```python
from build123d import *

# Parameters (mm, degrees)
SKETCH1_W                      = 60
SKETCH1_H                      = 120
BOSS_EXTRUDE1_DEPTH            = 80
CUT_EXTRUDE2_REACH             = 106.403
SKETCH3_W                      = 50.83
SKETCH3_H                      = 25.43
CUT_EXTRUDE2_DIRECTION_2_REACH = 106.403
CUT_EXTRUDE3_REACH             = 106.403
SKETCH5_W                      = 8.9675
SKETCH5_H                      = 100
CUT_EXTRUDE3_DIRECTION_2_REACH = 106.403
CUT_EXTRUDE4_REACH             = 106.403
SKETCH6_R                      = 6.365
CUT_EXTRUDE4_DIRECTION_2_REACH = 106.403
SKETCH7_W                      = 40.03
SKETCH7_H                      = 73
SKETCH7_R                      = 2.5
SKETCH7_W_2                    = 20.03
SKETCH7_H_2                    = 40.03
BOSS_EXTRUDE2_DEPTH            = 12.5
FILLET2_R                      = 5


with BuildPart() as part:
    # Sketch1 → Boss-Extrude1 (new, symmetric)
    with BuildSketch(Plane(origin=(0, 0, 0), x_dir=(1, 0, 0), z_dir=(0, 1, 0))):
        Rectangle(SKETCH1_W, SKETCH1_H)
    extrude(amount=BOSS_EXTRUDE1_DEPTH, both=True)

    # Cut-Extrude2: up to this face of the body (flat: up to its plane)
    cut_extrude2_end = Plane(part.part.faces().sort_by_distance((0, -80, 0))[0])
    # Sketch3 → Cut-Extrude2 (cut, up to the picked face)
    with BuildSketch(Plane(origin=(0, 0, 0), x_dir=(0, 0, -1), z_dir=(0, 1, 0)), mode=Mode.PRIVATE) as cut_extrude2_sk1:
        Rectangle(SKETCH3_W, SKETCH3_H)
    cut_extrude2_tool1 = split(extrude(cut_extrude2_sk1.sketch, amount=-CUT_EXTRUDE2_REACH, mode=Mode.PRIVATE), bisect_by=cut_extrude2_end, keep=Keep.BOTH, mode=Mode.PRIVATE)
    add(cut_extrude2_tool1.solids().sort_by(Axis((0, 0, 0), (0, -1, 0)))[0], mode=Mode.SUBTRACT)

    # Cut-Extrude2 direction 2: up to this face of the body (flat: up to its plane)
    cut_extrude2_direction_2_end = Plane(part.part.faces().sort_by_distance((0, 80, 0))[0])
    # Sketch3 → Cut-Extrude2 direction 2 (cut, up to the picked face)
    with BuildSketch(Plane(origin=(0, 0, 0), x_dir=(0, 0, -1), z_dir=(0, 1, 0)), mode=Mode.PRIVATE) as cut_extrude2_direction_2_sk1:
        Rectangle(SKETCH3_W, SKETCH3_H)
    cut_extrude2_direction_2_tool1 = split(extrude(cut_extrude2_direction_2_sk1.sketch, amount=CUT_EXTRUDE2_DIRECTION_2_REACH, mode=Mode.PRIVATE), bisect_by=cut_extrude2_direction_2_end, keep=Keep.BOTH, mode=Mode.PRIVATE)
    add(cut_extrude2_direction_2_tool1.solids().sort_by(Axis((0, 0, 0), (0, 1, 0)))[0], mode=Mode.SUBTRACT)

    # Cut-Extrude3: up to this face of the body (flat: up to its plane)
    cut_extrude3_end = Plane(part.part.faces().sort_by_distance((0, 0, 60))[0])
    # Sketch5 → Cut-Extrude3 (cut, up to the picked face)
    with BuildSketch(Plane.XY, mode=Mode.PRIVATE) as cut_extrude3_sk1:
        Rectangle(SKETCH5_W, SKETCH5_H)
    cut_extrude3_tool1 = split(extrude(cut_extrude3_sk1.sketch, amount=CUT_EXTRUDE3_REACH, mode=Mode.PRIVATE), bisect_by=cut_extrude3_end, keep=Keep.BOTH, mode=Mode.PRIVATE)
    add(cut_extrude3_tool1.solids().sort_by(Axis((0, 0, 0), (0, 0, 1)))[0], mode=Mode.SUBTRACT)

    # Cut-Extrude3 direction 2: up to this face of the body (flat: up to its plane)
    cut_extrude3_direction_2_end = Plane(part.part.faces().sort_by_distance((0, 0, -60))[0])
    # Sketch5 → Cut-Extrude3 direction 2 (cut, up to the picked face)
    with BuildSketch(Plane.XY, mode=Mode.PRIVATE) as cut_extrude3_direction_2_sk1:
        Rectangle(SKETCH5_W, SKETCH5_H)
    cut_extrude3_direction_2_tool1 = split(extrude(cut_extrude3_direction_2_sk1.sketch, amount=-CUT_EXTRUDE3_DIRECTION_2_REACH, mode=Mode.PRIVATE), bisect_by=cut_extrude3_direction_2_end, keep=Keep.BOTH, mode=Mode.PRIVATE)
    add(cut_extrude3_direction_2_tool1.solids().sort_by(Axis((0, 0, 0), (0, 0, -1)))[0], mode=Mode.SUBTRACT)

    # Cut-Extrude4: up to this face of the body (flat: up to its plane)
    cut_extrude4_end = Plane(part.part.faces().sort_by_distance((30, 0, 0))[0])
    # Sketch6 → Cut-Extrude4 (cut, up to the picked face)
    with BuildSketch(Plane(origin=(0, 0, 0), x_dir=(0, 0, -1), z_dir=(1, 0, 0)), mode=Mode.PRIVATE) as cut_extrude4_sk1:
        with Locations((-39.705, -30)):
            Circle(SKETCH6_R)
    cut_extrude4_tool1 = split(extrude(cut_extrude4_sk1.sketch, amount=CUT_EXTRUDE4_REACH, mode=Mode.PRIVATE), bisect_by=cut_extrude4_end, keep=Keep.BOTH, mode=Mode.PRIVATE)
    # Sketch6 → Cut-Extrude4 (cut, up to the picked face)
    with BuildSketch(Plane(origin=(0, 0, 0), x_dir=(0, 0, -1), z_dir=(1, 0, 0)), mode=Mode.PRIVATE) as cut_extrude4_sk2:
        with Locations((-39.705, 30)):
            Circle(SKETCH6_R)
    cut_extrude4_tool2 = split(extrude(cut_extrude4_sk2.sketch, amount=CUT_EXTRUDE4_REACH, mode=Mode.PRIVATE), bisect_by=cut_extrude4_end, keep=Keep.BOTH, mode=Mode.PRIVATE)
    # Sketch6 → Cut-Extrude4 (cut, up to the picked face)
    with BuildSketch(Plane(origin=(0, 0, 0), x_dir=(0, 0, -1), z_dir=(1, 0, 0)), mode=Mode.PRIVATE) as cut_extrude4_sk3:
        with Locations(Location((39.705, -30, 0), (0, 0, 180))):
            Circle(SKETCH6_R)
    cut_extrude4_tool3 = split(extrude(cut_extrude4_sk3.sketch, amount=CUT_EXTRUDE4_REACH, mode=Mode.PRIVATE), bisect_by=cut_extrude4_end, keep=Keep.BOTH, mode=Mode.PRIVATE)
    # Sketch6 → Cut-Extrude4 (cut, up to the picked face)
    with BuildSketch(Plane(origin=(0, 0, 0), x_dir=(0, 0, -1), z_dir=(1, 0, 0)), mode=Mode.PRIVATE) as cut_extrude4_sk4:
        with Locations(Location((39.705, 30, 0), (0, 0, 180))):
            Circle(SKETCH6_R)
    cut_extrude4_tool4 = split(extrude(cut_extrude4_sk4.sketch, amount=CUT_EXTRUDE4_REACH, mode=Mode.PRIVATE), bisect_by=cut_extrude4_end, keep=Keep.BOTH, mode=Mode.PRIVATE)
    add(cut_extrude4_tool1.solids().sort_by(Axis((0, -30, 39.705), (1, 0, 0)))[0], mode=Mode.SUBTRACT)
    add(cut_extrude4_tool2.solids().sort_by(Axis((0, 30, 39.705), (1, 0, 0)))[0], mode=Mode.SUBTRACT)
    add(cut_extrude4_tool3.solids().sort_by(Axis((0, -30, -39.705), (1, 0, 0)))[0], mode=Mode.SUBTRACT)
    add(cut_extrude4_tool4.solids().sort_by(Axis((0, 30, -39.705), (1, 0, 0)))[0], mode=Mode.SUBTRACT)

    # Cut-Extrude4 direction 2: up to this face of the body (flat: up to its plane)
    cut_extrude4_direction_2_end = Plane(part.part.faces().sort_by_distance((-30, 0, 0))[0])
    # Sketch6 → Cut-Extrude4 direction 2 (cut, up to the picked face)
    with BuildSketch(Plane(origin=(0, 0, 0), x_dir=(0, 0, -1), z_dir=(1, 0, 0)), mode=Mode.PRIVATE) as cut_extrude4_direction_2_sk1:
        with Locations((-39.705, -30)):
            Circle(SKETCH6_R)
    cut_extrude4_direction_2_tool1 = split(extrude(cut_extrude4_direction_2_sk1.sketch, amount=-CUT_EXTRUDE4_DIRECTION_2_REACH, mode=Mode.PRIVATE), bisect_by=cut_extrude4_direction_2_end, keep=Keep.BOTH, mode=Mode.PRIVATE)
    # Sketch6 → Cut-Extrude4 direction 2 (cut, up to the picked face)
    with BuildSketch(Plane(origin=(0, 0, 0), x_dir=(0, 0, -1), z_dir=(1, 0, 0)), mode=Mode.PRIVATE) as cut_extrude4_direction_2_sk2:
        with Locations((-39.705, 30)):
            Circle(SKETCH6_R)
    cut_extrude4_direction_2_tool2 = split(extrude(cut_extrude4_direction_2_sk2.sketch, amount=-CUT_EXTRUDE4_DIRECTION_2_REACH, mode=Mode.PRIVATE), bisect_by=cut_extrude4_direction_2_end, keep=Keep.BOTH, mode=Mode.PRIVATE)
    # Sketch6 → Cut-Extrude4 direction 2 (cut, up to the picked face)
    with BuildSketch(Plane(origin=(0, 0, 0), x_dir=(0, 0, -1), z_dir=(1, 0, 0)), mode=Mode.PRIVATE) as cut_extrude4_direction_2_sk3:
        with Locations(Location((39.705, -30, 0), (0, 0, 180))):
            Circle(SKETCH6_R)
    cut_extrude4_direction_2_tool3 = split(extrude(cut_extrude4_direction_2_sk3.sketch, amount=-CUT_EXTRUDE4_DIRECTION_2_REACH, mode=Mode.PRIVATE), bisect_by=cut_extrude4_direction_2_end, keep=Keep.BOTH, mode=Mode.PRIVATE)
    # Sketch6 → Cut-Extrude4 direction 2 (cut, up to the picked face)
    with BuildSketch(Plane(origin=(0, 0, 0), x_dir=(0, 0, -1), z_dir=(1, 0, 0)), mode=Mode.PRIVATE) as cut_extrude4_direction_2_sk4:
        with Locations(Location((39.705, 30, 0), (0, 0, 180))):
            Circle(SKETCH6_R)
    cut_extrude4_direction_2_tool4 = split(extrude(cut_extrude4_direction_2_sk4.sketch, amount=-CUT_EXTRUDE4_DIRECTION_2_REACH, mode=Mode.PRIVATE), bisect_by=cut_extrude4_direction_2_end, keep=Keep.BOTH, mode=Mode.PRIVATE)
    add(cut_extrude4_direction_2_tool1.solids().sort_by(Axis((0, -30, 39.705), (-1, 0, 0)))[0], mode=Mode.SUBTRACT)
    add(cut_extrude4_direction_2_tool2.solids().sort_by(Axis((0, 30, 39.705), (-1, 0, 0)))[0], mode=Mode.SUBTRACT)
    add(cut_extrude4_direction_2_tool3.solids().sort_by(Axis((0, -30, -39.705), (-1, 0, 0)))[0], mode=Mode.SUBTRACT)
    add(cut_extrude4_direction_2_tool4.solids().sort_by(Axis((0, 30, -39.705), (-1, 0, 0)))[0], mode=Mode.SUBTRACT)

    # Sketch7 → Boss-Extrude2 (add, symmetric)
    with BuildSketch(Plane(origin=(0, 0, 0), x_dir=(1, 0, 0), z_dir=(0, 1, 0))):
        with Locations((-50.015, 0)):
            Rectangle(SKETCH7_W, SKETCH7_H)
        with Locations(Location((-55.015, 24, 0), (0, 0, 270))):
            Circle(SKETCH7_R, mode=Mode.SUBTRACT)
        with Locations(Location((-45.015, 24, 0), (0, 0, 270))):
            Circle(SKETCH7_R, mode=Mode.SUBTRACT)
        with Locations(Location((-55.015, -24, 0), (0, 0, 270))):
            Circle(SKETCH7_R, mode=Mode.SUBTRACT)
        with Locations(Location((-45.015, -24, 0), (0, 0, 270))):
            Circle(SKETCH7_R, mode=Mode.SUBTRACT)
        with Locations((-50.015, 0)):
            Rectangle(SKETCH7_W_2, SKETCH7_H_2, mode=Mode.SUBTRACT)
    boss_extrude2 = extrude(amount=BOSS_EXTRUDE2_DEPTH, both=True)

    # Mirror2: Boss-Extrude2 across plane
    add(boss_extrude2.mirror(Plane(origin=(0, 0, 0), x_dir=(0, 0, 1), z_dir=(1, 0, 0))))

    # Fillet2
    fillet2_edges = [part.edges().sort_by_distance(p)[0] for p in [
        (-30, 12.5, 0),
        (-30, -12.5, 0),
        (-30, 0, 36.5),
        (-30, 0, -36.5),
        (-70.03, 0, -36.5),
        (-70.03, 0, 36.5),
        (30, 12.5, 0),
        (30, 0, -36.5),
        (30, 0, 36.5),
        (70.03, 0, 36.5),
        (70.03, 0, -36.5),
        (30, -12.5, 0),
    ]]
    fillet(fillet2_edges, radius=FILLET2_R)


solid = part.part
```
CAD build for the part. Positions are in the model's coordinates, mm. A direction names the side the tool comes from. Coordinates: 2 decimals unless noted, no trailing zeros. Order: outer loops, then holes, each group sorted by start corner. A loop starts at its lowest first (then second) coordinate and runs counter-clockwise, first axis right, second up. Notation, with made-up numbers: (9, -10.75) - (56, -10.75) arc R27 ccw to (56, 9.25) - close; hole circle Ø3 at (-17.75, -2.75). An arc over 180 degrees is marked (long way). Answer in a Markdown table with one row per item.
1. Slice it at D-D, the plane x = -0.5. List the corners of the cut face in (y, z) (3 decimals).
Answer:
| item | result |
|---|---|
| outline | (-80, -60) - (-50, -60) - (-50, -25.415) - (-80, -25.415) - close; (-80, 25.415) - (-50, 25.415) - (-50, 60) - (-80, 60) - close; (50, -60) - (80, -60) - (80, -25.415) - (50, -25.415) - close; (50, 25.415) - (80, 25.415) - (80, 60) - (50, 60) - close |
2. Slice it at C-C, the plane y = -30. Give the number of separate pieces and of enclosed holes in the cut face, then the cut area to 3 significant figures.
Answer:
| item | result |
|---|---|
| separate pieces | 6 |
| enclosed holes | 0 |
| area | 3,990 mm² |
3. 3-axis set-ups, long thin cutter, end or side, ignore diameter. For faces 4 (the face through (-50, 0, -20.015)), 5 (the face through (-50, 0, 36.5)), 6 (the face through (-4.484, -1, -42)): which of +Z, -Z, +X, -X, +Y, -Y reach the whole face in a straight line?
Answer:
| item | result |
|---|---|
| face 4 | +Y, -Y |
| face 5 | +Z, -X, +Y, -Y |
| face 6 | +Z, -Z |
4. Pull direction X, two halves, no side cores. Call faces 1 (the face through (31.43, -0.25, -38)), 2 (the face through (42.536, -0.175, -24.325)), 3 (the face through (-31.43, -0.25, -38)): +X half, -X half, draft (parallel to the pull), parting line (faces both ways), or undercut.
Answer:
| item | result |
|---|---|
| face 1 | +X half |
| face 2 | undercut |
| face 3 | -X half |
5. Slice it at B-B, the plane x = -18. List the corners of the cut face in (y, z) (3 decimals), then the cut area to 3 significant figures.
Answer:
| item | result |
|---|---|
| outline | (-80, -60) - (80, -60) - (80, 60) - (-80, 60) - close; hole circle Ø12.73 at (-30, -39.705); hole circle Ø12.73 at (-30, 39.705); hole circle Ø12.73 at (30, -39.705); hole circle Ø12.73 at (30, 39.705) |
| area | 18,700 mm² |
6. Slice it at A-A, the plane z = -8. List the corners of the cut face in (x, y) (3 decimals).
Answer:
| item | result |
|---|---|
| outline | (-70.03, -12.5) - (-60.03, -12.5) - (-60.03, 12.5) - (-70.03, 12.5) - close; (-40, -12.5) - (-35, -12.5) arc R5 cw to (-30, -17.5) - (-30, -80) - (-12.715, -80) - (-12.715, 80) - (-30, 80) - (-30, 17.5) arc R5 cw to (-35, 12.5) - (-40, 12.5) - close; (12.715, -80) - (30, -80) - (30, -17.5) arc R5 cw to (35, -12.5) - (40, -12.5) - (40, 12.5) - (35, 12.5) arc R5 cw to (30, 17.5) - (30, 80) - (12.715, 80) - close; (60.03, -12.5) - (70.03, -12.5) - (70.03, 12.5) - (60.03, 12.5) - close |
7. Drill centre lines: L1, parallel to X at y = 4.5, z = 24 (3 decimals); L2, parallel to X at y = 54.5, z = -20 (3 decimals); L3, parallel to Y at x = 28, z = 45. Where is each one in solid material? Low to high. Write a range as from..to.
Answer:
| item | result |
|---|---|
| L1 | -70.03..-57.515, -52.515..-47.515, -42.515..-12.715, 12.715..42.515, 47.515..52.515, 57.515..70.03 |
| L2 | -30..-12.715, 12.715..30 |
| L3 | -80..-33.53, -26.47..26.47, 33.53..80 |
8. Flat gauge pins, fed straight in: P1, Ø22, axis at x = -45.5, y = 2.5, coming from the +Z side; P2, Ø10, axis at y = 30, z = -39.705, coming from the -X side; P3, Ø6.5, axis at x = -45.015, z = 24, coming from the -Y side; P4, Ø20.5, axis at y = 30, z = 39.705, coming from the +X side. Where does each tip first touch, or does it go through?
Answer:
| item | result |
|---|---|
| P1 | z = 36.53 |
| P2 | through |
| P3 | y = -12.5 |
| P4 | x = 30 |
